Build history of the part. All positions in model axes, mm. Face numbers are marked on the shaded views. Coordinates: 2 decimals unless noted, no trailing zeros. Write each loop counter-clockwise with the first axis right and the second up, starting at its lowest first coordinate (ties: lowest second). Pieces come first, ordered by that corner, then holes.
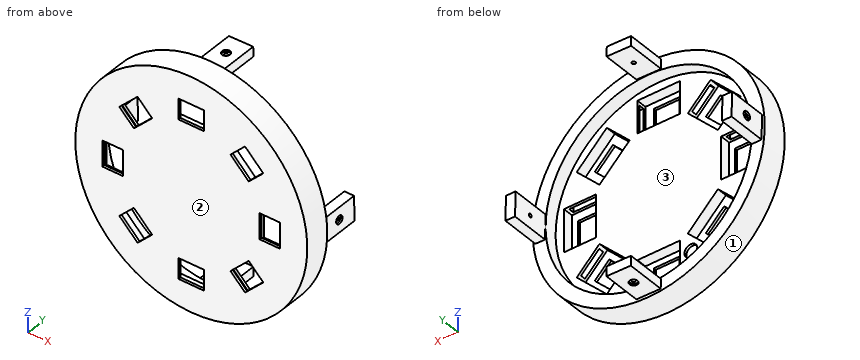
```python
from build123d import *

# Parameters (mm, degrees)
SKETCH2_R                                     = 45
BOSS_EXTRUDE1_DEPTH                           = 10
SKETCH3_R                                     = 40
CUT_EXTRUDE1_DEPTH                            = 5
SKETCH4_W                                     = 16.5
SKETCH4_H                                     = 12.5
SKETCH4_W_2                                   = 12.5
SKETCH4_H_2                                   = 16.5
CUT_EXTRUDE2_DEPTH                            = 4
SKETCH6_W                                     = 10
SKETCH6_H                                     = 8
CUT_EXTRUDE3_DEPTH                            = 65.272855857
CIRPATTERN1_COUNT                             = 8
SKETCH7_W                                     = 10
SKETCH7_H                                     = 2.006854622
CUT_REVOLVE1_ANGLE                            = 45
CIRPATTERN8_COUNT                             = 8
CUT_EXTRUDE4_REACH                            = 65.836
SKETCH10_R                                    = 2.5
BOSS_EXTRUDE2_DEPTH                           = 15
CIRPATTERN9_COUNT                             = 4
CBORE_START                                   = 40.100162841
CBORE_FOR_00_BINDING_HEAD_MACHINE_S_2_R       = 0.6985
CBORE_FOR_00_BINDING_HEAD_MACHINE_SCREW_DEPTH = 3.739789051
CBORE_START_2                                 = 43.128751892
CBORE_FOR_00_BINDING_HEAD_MACHINE_S_3_O_R     = 1.5875
CBORE_FOR_00_BINDING_HEAD_MACHINE_S_3_O_R_2   = 0.6985
CBORE_FOR_00_BINDING_HEAD_MACHINE_S_3_DEPTH   = 0.7112
CIRPATTERN10_COUNT                            = 4


# Read off the part's stored shape, not the designer's step: CBORE for #00 Binding Head Machine Screw3
with BuildPart() as part:
    # Sketch2 → Boss-Extrude1 (new body)
    with BuildSketch(Plane(origin=(0, 0, 0), x_dir=(1, 0, 0), z_dir=(0, 1, 0))):
        with Locations(Location((0, 0, 0), (0, 0, 270))):
            Circle(SKETCH2_R)
    extrude(amount=BOSS_EXTRUDE1_DEPTH)

    # Sketch3 → Cut-Extrude1 (cut)
    with BuildSketch(Plane(origin=(0, 10, 0), x_dir=(1, 0, 0), z_dir=(0, 1, 0))):
        with Locations(Location((0, 0, 0), (0, 0, 270))):
            Circle(SKETCH3_R)
    extrude(amount=-CUT_EXTRUDE1_DEPTH, mode=Mode.SUBTRACT)

    # Sketch4 → Cut-Extrude2 (cut)
    with BuildSketch(Plane(origin=(0, 5, 0), x_dir=(1, 0, 0), z_dir=(0, 1, 0))):
        with Locations((0, 30.477478673)):
            Rectangle(SKETCH4_W, SKETCH4_H)
        Polygon((20.136618281, 31.80388017), (11.297783516, 22.965045405), (22.965045405, 11.297783516), (31.80388017, 20.136618281), align=None)
        with Locations((30.477478673, 0)):
            Rectangle(SKETCH4_W_2, SKETCH4_H_2)
        Polygon((31.80388017, -20.136618281), (22.965045405, -11.297783516), (11.297783516, -22.965045405), (20.136618281, -31.80388017), align=None)
        with Locations((0, -30.477478673)):
            Rectangle(SKETCH4_W, SKETCH4_H)
        Polygon((-20.136618281, -31.80388017), (-11.297783516, -22.965045405), (-22.965045405, -11.297783516), (-31.80388017, -20.136618281), align=None)
        with Locations((-30.477478673, 0)):
            Rectangle(SKETCH4_W_2, SKETCH4_H_2)
        Polygon((-31.80388017, 20.136618281), (-22.965045405, 11.297783516), (-11.297783516, 22.965045405), (-20.136618281, 31.80388017), align=None)
    extrude(amount=-CUT_EXTRUDE2_DEPTH, mode=Mode.SUBTRACT)

    # Sketch6 → Cut-Extrude3 (cut, through all)
    with BuildSketch(Plane(origin=(0, 1, 0), x_dir=(1, 0, 0), z_dir=(0, 1, 0))):
        with Locations((0, 30.477478673)):
            Rectangle(SKETCH6_W, SKETCH6_H)
    cut_extrude3 = extrude(amount=-CUT_EXTRUDE3_DEPTH, mode=Mode.SUBTRACT)

    # CirPattern1: Cut-Extrude3 ×8 about axis
    cirpattern1_axis = Axis((0, 0, 0), (0, 1, 0))
    for i in range(1, CIRPATTERN1_COUNT):
        add(cut_extrude3.rotate(cirpattern1_axis, i * 360 / CIRPATTERN1_COUNT), mode=Mode.SUBTRACT)

    # Sketch7 → Cut-Revolve1 (revolve, cut)
    with BuildSketch(Plane(origin=(-8.25, 0, 0), x_dir=(0, 0, -1), z_dir=(1, 0, 0))):
        with Locations((30.477478673, 3)):
            Rectangle(SKETCH7_W, SKETCH7_H)
    cut_revolve1 = revolve(axis=Axis((-8.25, 5, -19.91726189), (0, 1, 0)), revolution_arc=CUT_REVOLVE1_ANGLE, mode=Mode.SUBTRACT)

    # CirPattern8: Cut-Revolve1 ×8 about axis
    cirpattern8_axis = Axis((0, 0, 0), (0, 1, 0))
    for i in range(1, CIRPATTERN8_COUNT):
        add(cut_revolve1.rotate(cirpattern8_axis, i * 360 / CIRPATTERN8_COUNT), mode=Mode.SUBTRACT)

    # Sketch10 → Cut-Extrude4 (cut, up to next)
    with BuildSketch(Plane(origin=(0, 5, 0), x_dir=(1, 0, 0), z_dir=(0, 1, 0)), mode=Mode.PRIVATE) as cut_extrude4_sk1:
        with Locations(Location((-12.45, 30.056958852, 0), (0, 0, 270))):
            Circle(SKETCH10_R)
    cut_extrude4_tool1 = extrude(cut_extrude4_sk1.sketch, amount=-CUT_EXTRUDE4_REACH, mode=Mode.PRIVATE) & part.part
    add(cut_extrude4_tool1.solids().sort_by_distance((-12.45, 5, -30.056959))[0], mode=Mode.SUBTRACT)

    # Sketch11 → Boss-Extrude2 (add)
    with BuildSketch(Plane(origin=(0, 10, 0), x_dir=(1, 0, 0), z_dir=(0, 1, 0))):
        Polygon((40.22065381, 4.733059783), (39.999995725, -4.78576812), (43.740789465, -4.78576812), (43.959438442, 4.646390178), align=None)
    boss_extrude2 = extrude(amount=BOSS_EXTRUDE2_DEPTH)

    # CirPattern9: Boss-Extrude2 ×4 about axis
    cirpattern9_axis = Axis((0, 0, 0), (0, 1, 0))
    for i in range(1, CIRPATTERN9_COUNT):
        add(boss_extrude2.rotate(cirpattern9_axis, i * 360 / CIRPATTERN9_COUNT))

    # CBORE for _00 Binding Head Machine S 2 → CBORE for #00 Binding Head Machine Screw3 (cut)
    with BuildSketch(Plane(origin=(0, 0, 0), x_dir=(0, 1, 0), z_dir=(0.9997314236585955, 0, 0.02317499837233911)).offset(CBORE_START)):
        with Locations((17.5, -0.946556065)):
            Circle(CBORE_FOR_00_BINDING_HEAD_MACHINE_S_2_R)
    cbore_for_00_binding_head_machine_screw = extrude(amount=CBORE_FOR_00_BINDING_HEAD_MACHINE_SCREW_DEPTH, mode=Mode.SUBTRACT)

    # CBORE for _00 Binding Head Machine S 3 o → CBORE for _00 Binding Head Machine S 3 (cut)
    with BuildSketch(Plane(origin=(0, 0, 0), x_dir=(0, 1, 0), z_dir=(0.9997314236585955, 0, 0.02317499837233911)).offset(CBORE_START_2)):
        with Locations((17.5, -0.946556065)):
            Circle(CBORE_FOR_00_BINDING_HEAD_MACHINE_S_3_O_R)
        with Locations((17.5, -0.946556065)):
            Circle(CBORE_FOR_00_BINDING_HEAD_MACHINE_S_3_O_R_2, mode=Mode.SUBTRACT)
    cbore_for_00_binding_head_machine_s_3 = extrude(amount=CBORE_FOR_00_BINDING_HEAD_MACHINE_S_3_DEPTH, mode=Mode.SUBTRACT)

    # CirPattern10: CBORE for #00 Binding Head Machine Screw3, CBORE for _00 Binding Head Machine S 3 ×4 about axis
    cirpattern10_axis = Axis((0, 0, 0), (0, 1, 0))
    add([cbore_for_00_binding_head_machine_screw.rotate(cirpattern10_axis, i * 360 / CIRPATTERN10_COUNT) for i in range(1, CIRPATTERN10_COUNT)], mode=Mode.SUBTRACT)
    add([cbore_for_00_binding_head_machine_s_3.rotate(cirpattern10_axis, i * 360 / CIRPATTERN10_COUNT) for i in range(1, CIRPATTERN10_COUNT)], mode=Mode.SUBTRACT)


solid = part.part
```
1. Saw through at D-D on y = 6.25. List the corners of the cut face in (x, z).
Computed values:
outline: circle Ø90 at (0, 0); hole circle Ø80 at (0, 0)
2. Saw through at A-A on y = 20.25. List the corners of the cut face in (x, z), plus the area to 3 significant figures.
Computed values:
outline: (-43.96, 4.65) - (-43.74, -4.79) - (-40, -4.79) - (-40.22, 4.73) - close; (-4.79, 40) - (4.73, 40.22) - (4.65, 43.96) - (-4.79, 43.74) - close; (-4.73, -40.22) - (-4.65, -43.96) - (4.79, -43.74) - (4.79, -40) - close; (40, 4.79) - (40.22, -4.73) - (43.96, -4.65) - (43.74, 4.79) - close
area: 142 mm2
3. Flat gauge pins, fed straight in: pin 1 (0.8 mm diameter, centred on y = 0.5, z = 2, fed in from -X); pin 2 (0.8 mm diameter, centred on x = 2, y = 0.5, fed in from +Z); pin 3 (10 mm diameter, centred on x = -1.5, z = 33.5, fed in from +Y). Where does each tip first touch, or does it go through?
Computed values:
pin 1: stops at x = -44.97
pin 2: stops at z = 44.97
pin 3: stops at y = 5
4. Mould opens along X. For the marked faces 1, 2 and 3 say: +X half, -X half, draft (parallel to the pull), parting line (faces both ways), or undercut.
Computed values:
face 1: parting line
face 2: draft
face 3: undercut
5. Saw through at B-B on z = -17. State how many separate pieces and enclosed holes the cut face has, plus the area to 3 significant figures.
Computed values:
separate pieces: 3
enclosed holes: 0
area: 356 mm2
6. Probe line 1 along X through (y, z) = (9, 0); line 2 along X through (y, z) = (2.25, -14); line 3 along Y through (x, z) = (22, -29). List the from-to ranges inside material, lowest first.
Computed values:
line 1: x = -45 to -40, 40 to 45
line 2: x = -42.77 to -34.38, -20.26 to 20.26, 34.38 to 42.77
line 3: y = 0 to 1
